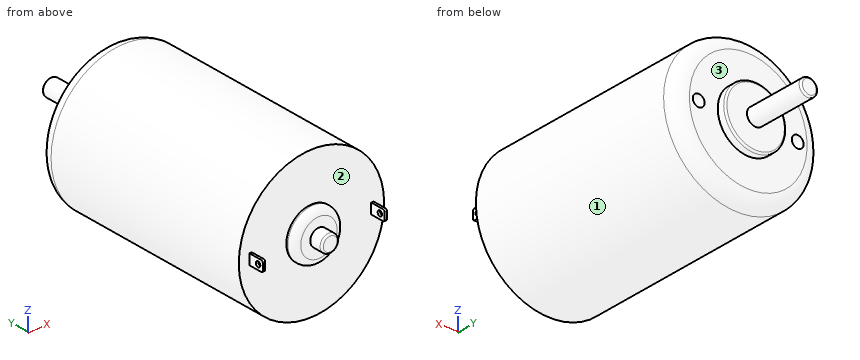
Solid Edge part; units mm, degrees
sketch "Sketch1" plane through (0, 0, 0) normal (0, -1, 0) x (1, 0, 0)
  circle A0 centre (0, 0) radius 21
extrude "Protrusion1" add sketch "Sketch1" along normal mid plane 67
fillet "Round_1" radius 4 1 edges at (-21, 33.5, 0)
sketch "Sketch2" plane through (0, 33.5, 0) normal (0, 1, 0) x (0, 0, -1)
  circle A0 centre (0, 0) radius 8.8
extrude "ExtrudedProtrusion_2" add sketch "Sketch2" along normal mid plane 5
sketch "Sketch3" plane through (0, 36, 0) normal (0, 1, 0) x (0, 0, -1)
  circle A0 centre (0, 0) radius 2.5
extrude "ExtrudedProtrusion_3" add sketch "Sketch3" along normal blind 18
fillet "Round_2" radius 0.5 2 edges at (0, 36, 8.8) (0, 54, 2.5)
sketch "Sketch4" plane through (0, 33.5, 0) normal (0, 1, 0) x (-1, 0, 0)
  circle A0 centre (14.3, 0) radius 1.7
  circle A1 centre (-14.3, 0) radius 1.7
extrude "ExtrudedCutout_1" cut sketch "Sketch4" against normal blind 12
sketch "Sketch5" plane through (0, -33.5, 0) normal (0, -1, 0) x (1, 0, 0)
  line L0 (17.25, -1.5) -> (17.95, -1.5)
  line L1 (17.95, -1.5) -> (17.95, 1.5)
  line L2 (17.95, 1.5) -> (17.25, 1.5)
  line L3 (17.25, 1.5) -> (17.25, -1.5)
  line L4 (-17.25, -1.5) -> (-17.95, -1.5)
  line L5 (-17.95, -1.5) -> (-17.95, 1.5)
  line L6 (-17.95, 1.5) -> (-17.25, 1.5)
  line L7 (-17.25, 1.5) -> (-17.25, -1.5)
extrude "ExtrudedProtrusion_4" add sketch "Sketch5" along normal mid plane 9
fillet "Round_3" radius 0.5 4 edges at (-17.6, -38, -1.5) (-17.6, -38, 1.5) (17.6, -38, -1.5) (17.6, -38, 1.5)
sketch "Sketch6" plane through (17.95, -35.75, 0) normal (1, 0, 0) x (0, 0, 1)
  circle A0 centre (0, 0.6716) radius 0.75
extrude "ExtrudedCutout_2" cut sketch "Sketch6" against normal blind 70
sketch "Sketch7" plane through (0, -33.5, 0) normal (0, -1, 0) x (0, 0, 1)
  circle A0 centre (0, 0) radius 7.25
extrude "ExtrudedProtrusion_5" add sketch "Sketch7" along normal mid plane 5
fillet "Round_4" radius 2 1 edges at (0, -36, -7.25)
sketch "Sketch8" plane through (0, -36, 0) normal (0, -1, 0) x (0, 0, 1)
  circle A0 centre (0, 0) radius 2.5
extrude "ExtrudedProtrusion_6" add sketch "Sketch8" along normal mid plane 7.6
fillet "Round_5" radius 0.5 1 edges at (0, -39.8, -2.5)
Read the model definition and answer for the solid it produces. Units are mm, in the model's axes. Face numbers are marked on the shaded views. A direction names the side the tool comes from. Round coordinates to 2 decimals unless told otherwise and drop trailing zeros. Loops run counter-clockwise (first coordinate to the right, second up) from the corner with the lowest first, then second, coordinate; pieces in that order, holes last. Notation, with made-up numbers: (-22, 81) - (26, 81) arc R20 ccw to (26, 109) - close; hole circle Ø9 at (-6.75, 33). An arc over 180 degrees is marked (long way). One line per question, with ' | ' between items. Start each with the question number.
Q1. Find the intervals of material crossed by L1, parallel to Y at x = -8.5, z = 4; L2, parallel to Z at x = 14, y = 26; L3, parallel to Z at x = 14.3, y = 25.25, in increasing order.
Q2. Section C-C on y = 25 is taken. Give the vertices of the cut face in (x, z), plus the area to 3 significant figures.
Q3. Section D-D on y = -5.5 is taken. Give the vertices of the cut face in (x, z), plus the area to 3 significant figures.
Q4. Section B-B on y = 45 is taken. Give the vertices of the cut face in (x, z).
Q5. For the marked faces 1, 2 and 3, determine the directions among +Z, -Z, +X, -X, +Y, -Y from which every point of the face is accessible in a straight line to the end or side of a thin tool.
Q6. Flat-ended cylindrical pins translate along their axes: pin 1 (1.5 mm diameter, centred on x = 4, z = 9, fed in from -Y); pin 2 (8 mm diameter, centred on y = -2.5, z = -1, fed in from +X); pin 3 (8 mm diameter, centred on x = -8, y = 27, fed in from -Z); pin 4 (3 mm diameter, centred on y = -4.5, z = -10, fed in from +X). Find the tip coordinate at first contact, or state that the pin passes through.
Established:
1) L1: -33.5 to 33.5 | L2: -15.65 to -1.67, 1.67 to 15.65 | L3: -15.38 to -1.7, 1.7 to 15.38
2) outline: circle Ø42 at (0, 0); hole circle Ø3.4 at (-14.3, 0); hole circle Ø3.4 at (14.3, 0) | area: 1,370 mm²
3) outline: circle Ø42 at (0, 0) | area: 1,390 mm²
4) outline: circle Ø5 at (0, 0)
5) face 1: +Y, -Y | face 2: -Y | face 3: +Y
6) pin 1: y = -33.5 | pin 2: x = 21 | pin 3: z = -20.62 | pin 4: x = 19.2
